Answer from the drawing. Dimensions are ordinates in mm from the lowest x, y and z of the part. Coordinates: 2 decimals unless noted, no trailing zeros. Write each loop counter-clockwise with the first axis right and the second up, starting at its lowest first coordinate (ties: lowest second). Pieces come first, ordered by that corner, then holes. Notation, with made-up numbers: (-17, 5.5) -> (-4, 5.5) arc R11 ccw to (-4, 23.5) -> close; hole circle Ø11 at (-2, -30). An arc over 180 degrees is marked (long way). One line per item, written item: value. Start each with the question number.
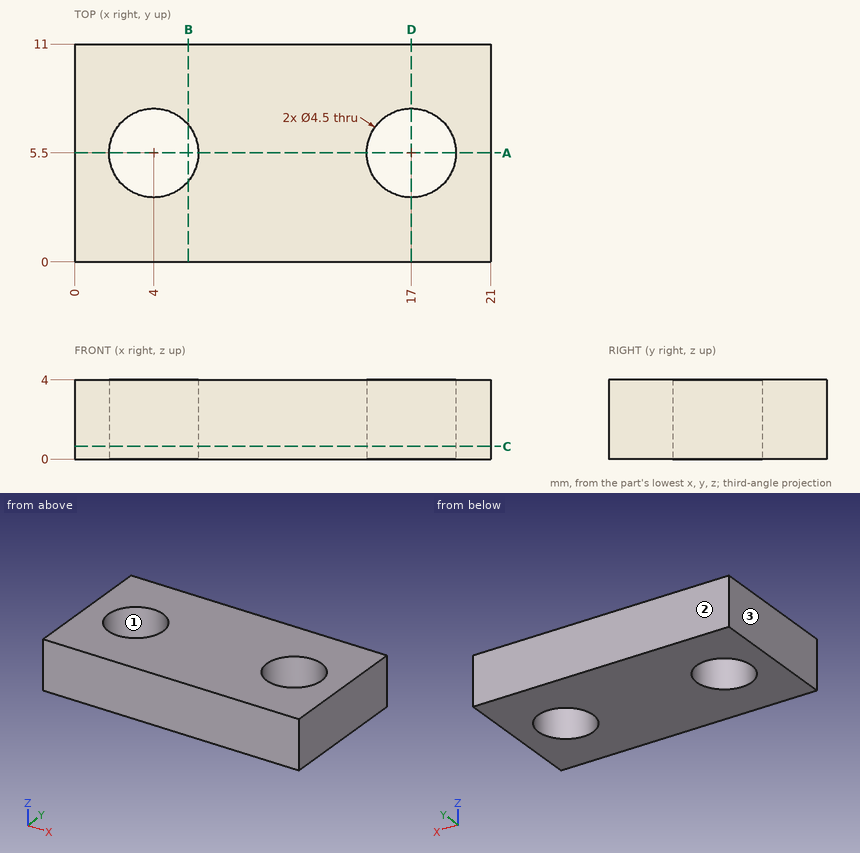
1. Given pin 1 (4 mm diameter, centred on x = 17, y = 5.5, fed in from -Z), flat-ended and moving along its own axis, determine where the tip first touches the part or whether it passes through.
2. Find the intervals of material crossed by probe 1 along X at (y, z) = (5.5, 3.1); probe 2 along Y at (x, z) = (4, 1.9); probe 3 along X at (y, z) = (6.5, 0.35), in increasing order. Write a range as from..to.
3. A cutting plane is placed at B-B on x = 5.75. Give the vertices of the cut face in (y, z), then the cut area to 3 significant figures.
4. For a pull along Y with two mould halves and no side action, classify the marked faces 1, 2 and 3 as +Y half, -Y half, draft (parallel to the pull), parting line (faces both ways), or undercut.
5. A cutting plane is placed at C-C on z = 0.65. Give the vertices of the cut face in (x, y).
6. A cutting plane is placed at D-D on x = 17. Give the vertices of the cut face in (y, z).
7. A cutting plane is placed at A-A on y = 5.5. Give the vertices of the cut face in (x, z), then the cut area to 3 significant figures.
Derived:
1. pin 1: passes through
2. probe 1: x = 0..1.75, 6.25..14.75, 19.25..21
2. probe 2: y = 0..3.25, 7.75..11
2. probe 3: x = 0..1.98, 6.02..14.98, 19.02..21
3. outline: (0, 0) -> (4.09, 0) -> (4.09, 4) -> (0, 4) -> close; (6.91, 0) -> (11, 0) -> (11, 4) -> (6.91, 4) -> close
3. area: 32.7 mm2
4. face 1: undercut
4. face 2: +Y half
4. face 3: draft
5. outline: (0, 0) -> (21, 0) -> (21, 11) -> (0, 11) -> close; hole circle Ø4.5 at (4, 5.5); hole circle Ø4.5 at (17, 5.5)
6. outline: (0, 0) -> (3.25, 0) -> (3.25, 4) -> (0, 4) -> close; (7.75, 0) -> (11, 0) -> (11, 4) -> (7.75, 4) -> close
7. outline: (0, 0) -> (1.75, 0) -> (1.75, 4) -> (0, 4) -> close; (6.25, 0) -> (14.75, 0) -> (14.75, 4) -> (6.25, 4) -> close; (19.25, 0) -> (21, 0) -> (21, 4) -> (19.25, 4) -> close
7. area: 48.0 mm2
